Source: three-view drawing plus pictorial views. Frame: mm from the lowest corner of the part. A direction names the side the tool comes from. Give positions to 0.01 mm unless a question says otherwise; leave off trailing zeros. Order: outer loops, then holes, each group sorted by start corner. A loop starts at its lowest first (then second) coordinate and runs counter-clockwise, first axis right, second up. Notation, with made-up numbers: (28, -23.75) - (41, -23.75) arc R10 cw to (41, -12.75) - close; hole circle Ø5 at (-0.5, 8). An arc over 180 degrees is marked (long way). Use one line per item in the form item = value.
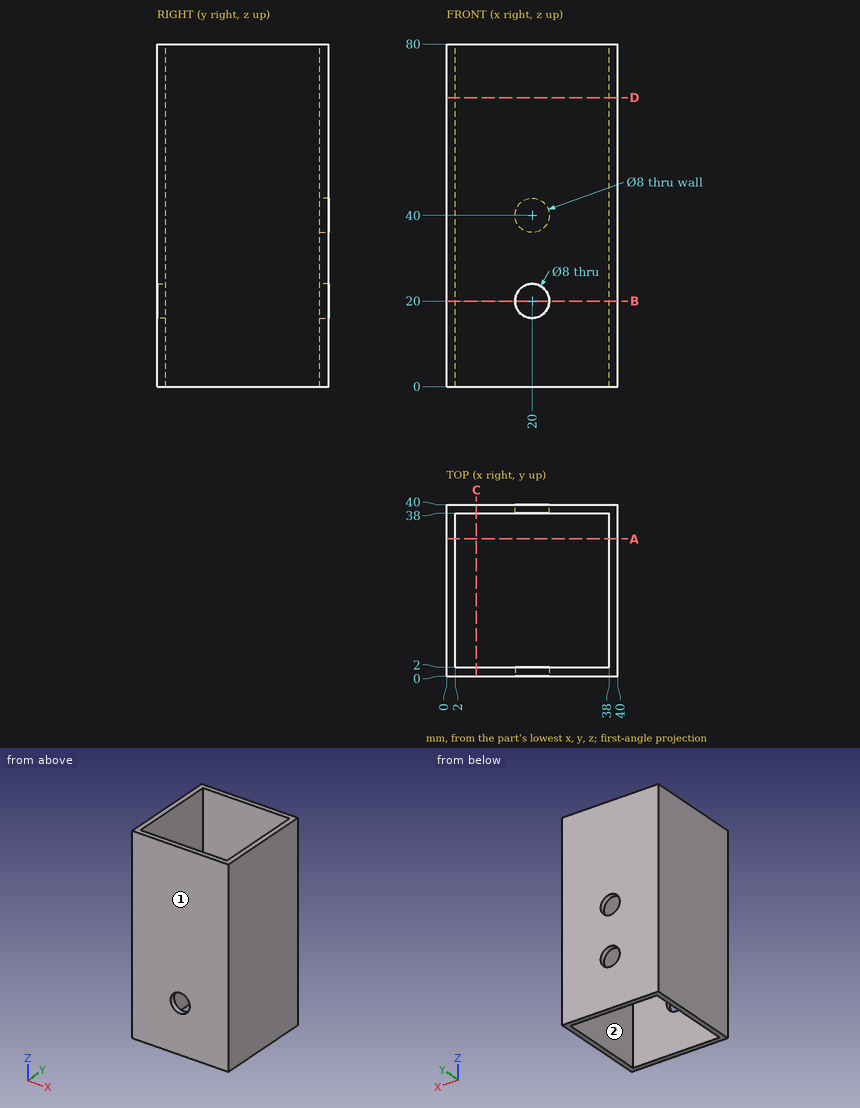
(1) Cut plane A-A on y = 32. Output: boundary loops of the cut face in (x, z).
Computed values:
outline = (0, 0) - (2, 0) - (2, 80) - (0, 80) - close; (38, 0) - (40, 0) - (40, 80) - (38, 80) - close
(2) Reachability of the marked faces 1 and 2 from +Z, -Z, +X, -X, +Y, -Y: full face, straight path, thin tool, end or side. Return the list, or none.
Computed values:
face_1 = +Z, -Z, +X, -X, -Y
face_2 = +Z, -Z
(3) Cut plane B-B on z = 20. Output: boundary loops of the cut face in (x, y).
Computed values:
outline = (0, 0) - (16, 0) - (16, 2) - (2, 2) - (2, 38) - (16, 38) - (16, 40) - (0, 40) - close; (24, 0) - (40, 0) - (40, 40) - (24, 40) - (24, 38) - (38, 38) - (38, 2) - (24, 2) - close
(4) Cut plane D-D on z = 67.5. Output: boundary loops of the cut face in (x, y).
Computed values:
outline = (0, 0) - (40, 0) - (40, 40) - (0, 40) - close; hole (2, 2) - (38, 2) - (38, 38) - (2, 38) - close
(5) Ray query, line 1 along Y through (x, z) = (9.5, 48.5); line 2 along X through (y, z) = (38.65, 40). Return the intervals inside material, ascending.
Computed values:
line_1 = 0 to 2, 38 to 40
line_2 = 0 to 16, 24 to 40
